from build123d import *

# Parameters (mm, degrees)
F0_W     = 50.8
F0_H     = 38.1
F1_DEPTH = 31.75
F3_DEPTH = 254
F4_W     = 25.4
F4_H     = 19.05
F5_DEPTH = 25.4


with BuildPart() as f1:
    # F0 (on Front) → F1 (new body)
    with BuildSketch(Plane.XZ):
        with Locations((14.420407, 5.444671)):
            Rectangle(F0_W, F0_H)
    extrude(amount=F1_DEPTH)

    # F2 (on face) → F3 (cut)
    with BuildSketch(Plane.YZ.offset(39.820407)):
        with BuildLine():
            ThreePointArc((-30.30265, -0.864059), (-22.096181, 1.000761), (-14.949479, 5.444671))
            ThreePointArc((-14.949479, 5.444671), (-8.599479, 14.04415), (-6.35, 24.494671))
            Line((-6.35, 24.494671), (-31.75, 24.494671))
            Line((-31.75, 24.494671), (-31.75, -0.905329))
            Line((-31.75, -0.905329), (-30.30265, -0.864059))
        make_face()
    extrude(amount=-F3_DEPTH, mode=Mode.SUBTRACT)

    # F4 (on face) → F5 (cut)
    with BuildSketch(Plane(origin=(0, 0, 0), x_dir=(-1, 0, 0), z_dir=(0, 1, 0))):
        with Locations((-14.420407, 14.969671)):
            Rectangle(F4_W, F4_H)
    extrude(amount=-F5_DEPTH, mode=Mode.SUBTRACT)


solid = f1.part
For this review, take the finished solid that the model builds, in its own axes (mm). A direction names the side the tool comes from. Coordinates: 2 decimals unless noted, no trailing zeros. Order: outer loops, then holes, each group sorted by start corner. A loop starts at its lowest first (then second) coordinate and runs counter-clockwise, first axis right, second up. Notation, with made-up numbers: (39, 56) -> (78, 56) arc R28 ccw to (78, 95) -> close; hole circle Ø11 at (88, -28.75). An arc over 180 degrees is marked (long way). Return JSON: item names as keys, results as strings.
1. We need section C-C on y = -4. Write out the cut boundary in (x, z).
Answer block:
{"outline": "(-10.98, -13.61) -> (39.82, -13.61) -> (39.82, 24.49) -> (27.12, 24.49) -> (27.12, 5.44) -> (1.72, 5.44) -> (1.72, 24.49) -> (-10.98, 24.49) -> close"}
2. For line 1 (X direction, y = -9, z = 5.5); line 2 (Z direction, x = 19, y = -14); line 3 (Z direction, x = 31, y = -25), list the stretches that pass through material, from the lowest coordinate up. Write a range as from..to.
Answer block:
{"line 1": "-10.98..1.72, 27.12..39.82", "line 2": "-13.61..5.44", "line 3": "-13.61..0.01"}
3. The part is to be moulded in two halves that separate along X. For faces 3 (the flat face through (-10.98, -12, 1)), 4 (the flat face through (-5, -3, 24.495)), 5 (the flat face through (27.12, -4, 13)), say which applies: +X half, -X half, draft (parallel to the pull), parting line (faces both ways), or undercut.
Answer block:
{"face 3": "-X half", "face 4": "draft", "face 5": "undercut"}
4. We need section A-A on z = 18. Write out the cut boundary in (x, y).
Answer block:
{"outline": "(-10.98, -7.19) -> (1.72, -7.19) -> (1.72, 0) -> (-10.98, 0) -> close; (27.12, -7.19) -> (39.82, -7.19) -> (39.82, 0) -> (27.12, 0) -> close"}
5. Machinability: for faces 1 (the flat face through (1.72, -4, 13)), 2 (the flat face through (14, -16, -13.605)), which of the approach directions +Z, -Z, +X, -X, +Y, -Y give a long, thin tool a straight path to every point of the face, cutting with its end or side? Answer none if there is none.
Answer block:
{"face 1": "+Z, +Y, -Y", "face 2": "-Z, +X, -X, +Y, -Y"}
6. We need section B-B on x = 36. Write out the cut boundary in (y, z).
Answer block:
{"outline": "(-31.75, -13.61) -> (0, -13.61) -> (0, 24.49) -> (-6.35, 24.49) arc R25.4 cw to (-14.95, 5.44) arc R25.4 cw to (-30.3, -0.86) -> (-31.75, -0.91) -> close"}
7. We need section D-D on z = 7.5. Write out the cut boundary in (x, y), and give its area (3 significant figures).
Answer block:
{"outline": "(-10.98, -12.87) -> (1.72, -12.87) -> (1.72, 0) -> (-10.98, 0) -> close; (27.12, -12.87) -> (39.82, -12.87) -> (39.82, 0) -> (27.12, 0) -> close", "area": "327 mm²"}
8. For pin 1 Ø10 at (y, z) = (-15, 19.5) entering from -X; pin 2 Ø12 at (x, y) = (9, -5) entering from +Z; pin 3 Ø12 at (x, y) = (2.5, -18.5) entering from +Z, all flat-tipped, find the tip position at first contact; note any pin that passes through.
Answer block:
{"pin 1": "through", "pin 2": "z = 5.44", "pin 3": "z = 7.86"}
